Geometry: see drawing. Coordinates: mm, zero at the bounding-box minimum. Coordinates: 2 decimals unless noted, no trailing zeros. Write each loop counter-clockwise with the first axis right and the second up, starting at its lowest first coordinate (ties: lowest second). Pieces come first, ordered by that corner, then holes. Notation, with made-up numbers: (-5.75, 43) -> (0.25, 43) arc R24 ccw to (0.25, 55) -> close; hole circle Ø1 at (58, -21). An arc over 180 degrees is marked (long way). Use one line per item in the form item = value. Start each with the question number.
(1) Cut plane B-B on x = 19. Return the cut outline in (y, z).
(2) First-contact query: pin 1 (0.6 mm diameter, centred on y = 1.5, z = 1, fed in from +X); pin 2 (1.3 mm diameter, centred on x = 19.5, z = 0.5, fed in from -Y); pin 3 (10 mm diameter, centred on x = 22.5, z = 17.5, fed in from -Y); pin 4 (10.5 mm diameter, centred on x = 4, z = 15.5, fed in from -Y). Flat tips, straight axial feed; report the tip coordinate or a pass-through.
(3) Cut plane A-A on y = 2.5. Return the cut outline in (x, z), plus the area to 3 significant figures.
(4) Cut plane D-D on y = 8. Return the cut outline in (x, z).
(5) Pull-direction query (X, two-part tool) for the marked faces 1, 2 and 3; classes: released by +X, released by -X, zero draft, split by the parting line, or undercut.
(6) Cut plane C-C on z = 14. Return the cut outline in (x, y).
(7) Ray query, line 1 along X through (y, z) = (8.5, 24.5); line 2 along Y through (x, z) = (29, 32); line 3 along Z through (x, y) = (16.5, 1.5). Return the intervals inside material, ascending.
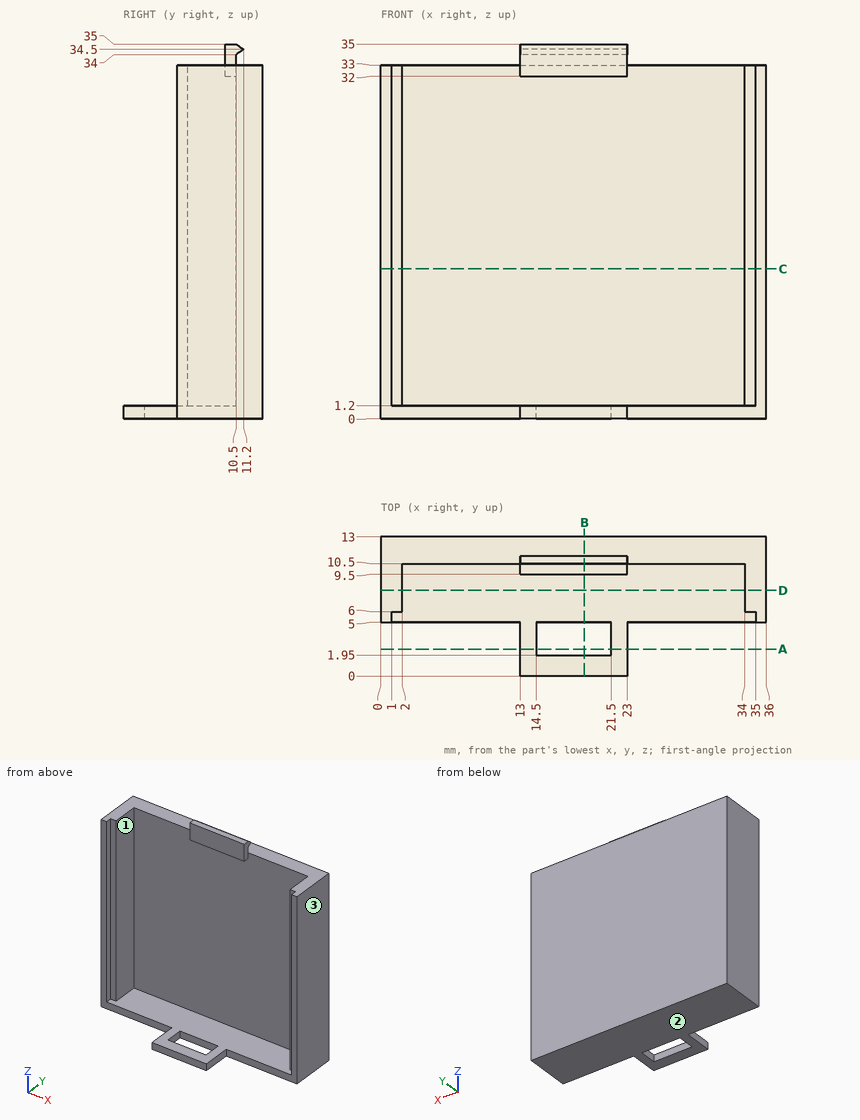
Values:
q1.outline = (0, 0) -> (1.95, 0) -> (1.95, 1.2) -> (0, 1.2) -> close; (5, 0) -> (13, 0) -> (13, 33) -> (10.5, 33) -> (10.5, 34) -> (11.2, 34.5) -> (10.5, 35) -> (9.5, 35) -> (9.5, 32) -> (10.5, 32) -> (10.5, 1.2) -> (5, 1.2) -> close
q2.pin_1 = 23
q2.pin_2 = 0
q2.pin_3 = 10.5
q2.pin_4 = 5
q3.outline = (13, 0) -> (14.5, 0) -> (14.5, 1.2) -> (13, 1.2) -> close; (21.5, 0) -> (23, 0) -> (23, 1.2) -> (21.5, 1.2) -> close
q3.area = 3.60 mm2
q4.outline = (0, 0) -> (36, 0) -> (36, 33) -> (34, 33) -> (34, 1.2) -> (2, 1.2) -> (2, 33) -> (0, 33) -> close
q5.face_1 = undercut
q5.face_2 = zero draft
q5.face_3 = released by +X
q6.outline = (0, 5) -> (1, 5) -> (1, 6) -> (2, 6) -> (2, 10.5) -> (34, 10.5) -> (34, 6) -> (35, 6) -> (35, 5) -> (36, 5) -> (36, 13) -> (0, 13) -> close
q7.line_1 = 0 to 2, 34 to 36
q7.line_2 = 10.5 to 13
q7.line_3 = 0 to 1.2
